Geometry: final body of the model. Coordinates: model frame, mm. A direction names the side the tool comes from. Coordinates: 2 decimals unless noted, no trailing zeros. Order: outer loops, then holes, each group sorted by start corner. A loop starts at its lowest first (then second) coordinate and runs counter-clockwise, first axis right, second up. Notation, with made-up numbers: M 24,73 L 33,73 A7 ccw 33,85 Z; hole C 47.25,-33 d9. An arc over 180 degrees is marked long. Write item = value, one per line. Start each with the question number.
```python
from build123d import *

# Parameters (mm, degrees)
F0_W     = 40
F0_H     = 40
F1_DEPTH = 60
F2_W     = 34
F2_H     = 54
F3_DEPTH = 37
F4_W     = 20
F4_H     = 30
F5_DEPTH = 40.001
F6_W     = 10
F6_H     = 30
F7_DEPTH = 3


with BuildPart() as f1:
    # F0 (on Front) → F1 (new body)
    with BuildSketch(Plane.XZ):
        Rectangle(F0_W, F0_H)
    extrude(amount=F1_DEPTH)

    # F2 (on face) → F3 (cut, through all)
    with BuildSketch(Plane.XY.offset(20)):
        with Locations((0, -30)):
            Rectangle(F2_W, F2_H)
    extrude(amount=-F3_DEPTH, mode=Mode.SUBTRACT)

    # F4 (on face) → F5 (cut, through all)
    with BuildSketch(Plane.YZ.offset(20)):
        with Locations((-30, 5)):
            Rectangle(F4_W, F4_H)
    extrude(amount=-F5_DEPTH, mode=Mode.SUBTRACT)

    # F6 (on face) → F7 (cut, through all)
    with BuildSketch(Plane.XZ.offset(60)):
        with Locations((0, 5)):
            Rectangle(F6_W, F6_H)
    extrude(amount=-F7_DEPTH, mode=Mode.SUBTRACT)


solid = f1.part
```
Item 1: Material intervals for probe 1 along X at (y, z) = (-42.5, -12.5); probe 2 along Y at (x, z) = (1, -13.5); probe 3 along Y at (x, z) = (18, 9), sorted ascending. Write a range as [from, to].
Item 2: Section query B-B on x = -3. Output: boundary loops of the cut face in (y, z).
Item 3: Section query C-C on y = -19. Output: boundary loops of the cut face in (x, z).
Item 4: Section query A-A on z = 3. Output: boundary loops of the cut face in (x, y).
Item 5: Draft query along Y for faces 5 (the flat face through (0, 0, 0)), 6 (the flat face through (-18, -40, 5)), 7 (the flat face through (0, -59, -10)), 8 (the flat face through (19, -40, 5)). Return one class per face: pulls with the +Y half, pulls with the -Y half, needs draft (parallel to the pull), parting line crosses it, or undercut.
Item 6: First-contact query: pin 1 (3.5 mm diameter, centred on x = -18, y = -26.5, fed in from +Z); pin 2 (5 mm diameter, centred on x = -13, y = -26.5, fed in from +Z). Flat tips, straight axial feed; report the tip coordinate or a pass-through.
Item 7: Reachability of faces 1 (the flat face through (-18, -20, 5)), 2 (the flat face through (0, -3, 2)), 3 (the flat face through (-5, -59, 5)), 4 (the flat face through (-0.1, -2.5, 20)) from +Z, -Z, +X, -X, +Y, -Y: full face, straight path, thin tool, end or side. Return the list, or none.
Ans:
q1.probe_1 = [-20, -17], [17, 20]
q1.probe_2 = [-60, -57], [-3, 0]
q1.probe_3 = [-60, -40], [-20, 0]
q2.outline = M -60,-20 L 0,-20 L 0,20 L -3,20 L -3,-17 L -57,-17 L -57,-10 L -60,-10 Z
q3.outline = M -20,-20 L 20,-20 L 20,20 L 17,20 L 17,-17 L -17,-17 L -17,20 L -20,20 Z
q4.outline = M -20,-60 L -5,-60 L -5,-57 L -17,-57 L -17,-40 L -20,-40 Z; M -20,-20 L -17,-20 L -17,-3 L 17,-3 L 17,-20 L 20,-20 L 20,0 L -20,0 Z; M 5,-60 L 20,-60 L 20,-40 L 17,-40 L 17,-57 L 5,-57 Z
q5.face_5 = pulls with the +Y half
q5.face_6 = undercut
q5.face_7 = needs draft
q5.face_8 = undercut
q6.pin_1 = -10
q6.pin_2 = -17
q7.face_1 = +Z, +X, -X
q7.face_2 = +Z
q7.face_3 = +Z, -Y
q7.face_4 = +Z, +X, -X, +Y, -Y
